Here's how the part is built. I have some questions about the finished solid (model axes, mm). Face numbers are marked on the shaded views. A direction names the side the tool comes from. Coordinates: 2 decimals unless noted, no trailing zeros. Write each loop counter-clockwise with the first axis right and the second up, starting at its lowest first coordinate (ties: lowest second). Pieces come first, ordered by that corner, then holes. Notation, with made-up numbers: (2.5, 58.5) -> (47.5, 58.5) arc R34 cw to (47.5, 90.5) -> close; hole circle Ø8 at (-3, -27.5). An arc over 180 degrees is marked (long way). Put each result on its own line as item: value. Start each with the question number.
Item 1: If we mould it in two halves opening along Y, with no side actions, what happens to the marked faces 6, 7, 8 and 9? For each: released by +Y, released by -Y, zero draft, split by the parting line, or undercut.
Item 2: I need wall thicknesses on line 1 (Y direction, x = -12.75, z = -3.5); line 2 (Y direction, x = -15.75, z = -1.5); line 3 (Z direction, x = -14, y = 3.75). Which ranges of each line are inside material? Lowest first, please. Write a range as [from, to].
Item 3: On a 3-axis mill with a long thin cutter (end or side, diameter ignored), from which of +Z, -Z, +X, -X, +Y, -Y can I reach the whole of each face in a straight line? I mean the marked faces 1, 2, 3, 4 and 5. Say none if no direction works.
Item 4: I want a section at C-C, the plane y = -5.75. List the corners of the cut face in (x, z) for me, then the cut area to 3 significant figures.
Item 5: I want a section at D-D, the plane x = -10.5. List the corners of the cut face in (y, z) for me (3 decimals).
Item 6: I want a section at A-A, the plane x = -15. List the corners of the cut face in (y, z) for me (3 decimals).
Item 7: For pin 1 (0.7 mm diameter, centred on y = -8.5, z = -2.5, fed in from -X); pin 2 (0.5 mm diameter, centred on y = -4.5, z = 3.5, fed in from -X); pin 3 (2 mm diameter, centred on y = 4.5, z = 1, fed in from -X), each with a flat end and sliding along its axis, tell me the tip position at first contact or that it passes through.
Item 8: I want a section at B-B, the plane z = -2.25. List the corners of the cut face in (x, y) for me, then the cut area to 3 significant figures.
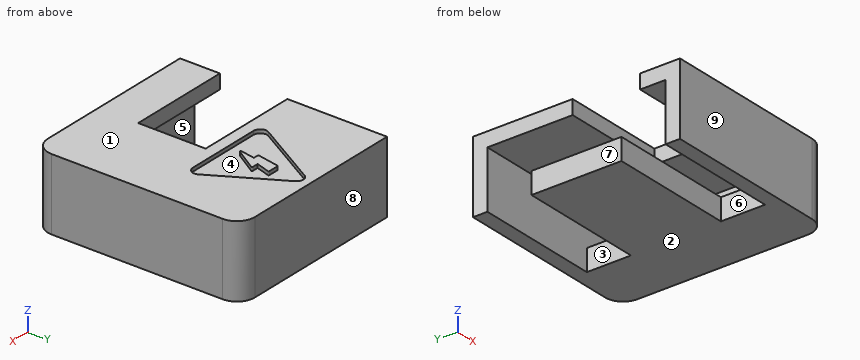
from build123d import *

# Parameters (mm, degrees)
ESQUISSE1_W             = 8
ESQUISSE1_H             = 23
BOSS_EXTRU_1_DEPTH      = 1.6
ESQUISSE2_W             = 2.4
ESQUISSE2_H             = 10
BOSS_EXTRU_2_DEPTH      = 19
ESQUISSE3_W             = 2.4
ESQUISSE3_H             = 19.8
BOSS_EXTRU_3_DEPTH      = 5
ENL_V_MAT_EXTRU_1_REACH = 25.606
ESQUISSE4_W             = 11.5
ESQUISSE4_H             = 7.5
ENL_V_START             = -0.4
ENL_V_MAT_EXTRU_2_DEPTH = 0.4
CONG_1_R                = 2


# Read off the part's stored shape, not the designer's step: Enlèv. mat.-Extru.2
with BuildPart() as part:
    # Esquisse1 → Boss.-Extru.1 (new body)
    with BuildSketch(Plane(origin=(0, 0, 0), x_dir=(0, 0, -1), z_dir=(1, 0, 0))):
        Rectangle(ESQUISSE1_W, ESQUISSE1_H)
    extrude(amount=BOSS_EXTRU_1_DEPTH)

    # Esquisse2 → Boss.-Extru.2 (add)
    with BuildSketch(Plane.ZY):
        Polygon((-4, 11.5), (4, 11.5), (4, -11.5), (-4, -11.5), (-4, -9.9), (2.4, -9.9), (2.4, 9.9), (-4, 9.9), align=None)
        with Locations((-2.8, 0)):
            Rectangle(ESQUISSE2_W, ESQUISSE2_H)
    extrude(amount=BOSS_EXTRU_2_DEPTH)

    # Esquisse3 → Boss.-Extru.3 (add)
    with BuildSketch(Plane.ZY):
        with Locations((-2.8, 0)):
            Rectangle(ESQUISSE3_W, ESQUISSE3_H)
    extrude(amount=BOSS_EXTRU_3_DEPTH)

    # Esquisse4 → Enlèv. mat.-Extru.1 (cut, up to next)
    with BuildSketch(Plane.XY.offset(4), mode=Mode.PRIVATE) as enl_v_mat_extru_1_sk1:
        with Locations((-13.25, -3.325)):
            Rectangle(ESQUISSE4_W, ESQUISSE4_H)
    enl_v_mat_extru_1_tool1 = extrude(enl_v_mat_extru_1_sk1.sketch, amount=-ENL_V_MAT_EXTRU_1_REACH, mode=Mode.PRIVATE) & part.part
    add(enl_v_mat_extru_1_tool1.solids().sort_by_distance((-13.25, -3.325, 4))[0], mode=Mode.SUBTRACT)

    # Enlèv. mat.-Extru.2 outline → Enlèv. mat.-Extru.2 (cut)
    with BuildSketch(Plane.XY.offset(4).offset(ENL_V_START)):
        with BuildLine():
            Line((-12.608271193, 1.69730271), (-4.088687559, 1.69730271))
            add(Edge.make_bspline(
                [(-4.088687559, 1.69730271), (-3.506604225, 1.697303518), (-3.136187559, 2.332303518), (-3.432521215, 2.840303033)],
                knots=[5, 5, 5, 5, 6, 6, 6, 6], degree=3))
            Line((-3.432521215, 2.840303033), (-7.687021295, 10.227470021))
            add(Edge.make_bspline(
                [(-7.687021295, 10.227470021), (-7.983354547, 10.735470041), (-8.713604709, 10.735470041), (-9.009937961, 10.227470021)],
                knots=[1, 1, 1, 1, 2, 2, 2, 2], degree=3))
            Line((-9.009937961, 10.227470021), (-13.275021213, 2.840303033))
            add(Edge.make_bspline(
                [(-13.275021213, 2.840303033), (-13.571354541, 2.33230271), (-13.200937899, 1.69730271), (-12.608271193, 1.69730271)],
                knots=[3, 3, 3, 3, 4, 4, 4, 4], degree=3))
        make_face()
        with BuildLine():
            add(Edge.make_bspline(
                [(-7.380104467, 5.570803355), (-7.337771376, 5.623720022), (-7.380104467, 5.708386608), (-7.454188284, 5.708387012)],
                knots=[11, 11, 11, 11, 12, 12, 12, 12], degree=3))
            Line((-7.380104467, 5.570803355), (-8.9146878, 3.115470345))
            add(Edge.make_bspline(
                [(-9.0734378, 3.178970184), (-9.094604547, 3.083720023), (-8.967604466, 3.030803356), (-8.9146878, 3.115470345)],
                knots=[1, 1, 1, 1, 2, 2, 2, 2], degree=3))
            Line((-9.0734378, 3.178970184), (-8.787687719, 4.766470184))
            Line((-8.787687719, 4.766470184), (-9.306271214, 4.766470184))
            add(Edge.make_bspline(
                [(-9.390937799, 4.872303517), (-9.401521375, 4.81938685), (-9.35918788, 4.766470184), (-9.306271214, 4.766470184)],
                knots=[4, 4, 4, 4, 5, 5, 5, 5], degree=3))
            Line((-9.390937799, 4.872303517), (-8.957021294, 7.253553516))
            add(Edge.make_bspline(
                [(-8.872354708, 7.32763693), (-8.9146878, 7.32763693), (-8.946438123, 7.295887011), (-8.957021294, 7.253553516)],
                knots=[6, 6, 6, 6, 7, 7, 7, 7], degree=3))
            Line((-8.872354708, 7.32763693), (-7.739937961, 7.32763693))
            add(Edge.make_bspline(
                [(-7.655271375, 7.211220425), (-7.634104628, 7.274720264), (-7.676438123, 7.32763693), (-7.739937961, 7.32763693)],
                knots=[8, 8, 8, 8, 9, 9, 9, 9], degree=3))
            Line((-7.655271375, 7.211220425), (-8.120938204, 5.708387012))
            Line((-8.120938204, 5.708387012), (-7.454188284, 5.708387012))
        make_face(mode=Mode.SUBTRACT)
    extrude(amount=ENL_V_MAT_EXTRU_2_DEPTH, mode=Mode.SUBTRACT)

    # Congé1
    cong_1_edges = [part.edges().sort_by_distance(p)[0] for p in [
        (1.6, -11.5, 0),
        (1.6, 11.5, 0),
    ]]
    fillet(cong_1_edges, radius=CONG_1_R)


solid = part.part
Calculated:
1. face 6: undercut
1. face 7: zero draft
1. face 8: released by +Y
1. face 9: released by -Y
2. line 1: y = [-11.5, -9.9], [-5, 5], [9.9, 11.5]
2. line 2: y = [-11.5, -9.9], [9.9, 11.5]
2. line 3: z = [-4, -1.6], [2.4, 4]
3. face 1: +Z, +X, -X, +Y, -Y
3. face 2: -Z, +X, -X, +Y, -Y
3. face 3: -Z, -X
3. face 4: +Z
3. face 5: -X
4. outline: (-7.5, 2.4) -> (0, 2.4) -> (0, -1.6) -> (-5, -1.6) -> (-5, -4) -> (1.6, -4) -> (1.6, 4) -> (-7.5, 4) -> close
4. area: 36.8 mm2
5. outline: (-11.5, -4) -> (-9.9, -4) -> (-9.9, 2.4) -> (-7.075, 2.4) -> (-7.075, 4) -> (-11.5, 4) -> close; (-5, -4) -> (5, -4) -> (5, -1.6) -> (-5, -1.6) -> close; (0.425, 2.4) -> (9.9, 2.4) -> (9.9, -4) -> (11.5, -4) -> (11.5, 4) -> (7.647, 4) -> (7.647, 3.6) -> (1.697, 3.6) -> (1.697, 4) -> (0.425, 4) -> close
6. outline: (-11.5, -4) -> (-9.9, -4) -> (-9.9, 2.4) -> (-7.075, 2.4) -> (-7.075, 4) -> (-11.5, 4) -> close; (-5, -4) -> (5, -4) -> (5, -1.6) -> (-5, -1.6) -> close; (0.425, 2.4) -> (9.9, 2.4) -> (9.9, -4) -> (11.5, -4) -> (11.5, 4) -> (0.425, 4) -> close
7. pin 1: stops at x = -5
7. pin 2: stops at x = -7.5
7. pin 3: stops at x = 0
8. outline: (-19, -11.5) -> (-0.4, -11.5) arc R2 ccw to (1.6, -9.5) -> (1.6, 9.5) arc R2 ccw to (-0.4, 11.5) -> (-19, 11.5) -> (-19, 9.9) -> (-5, 9.9) -> (-5, 5) -> (-19, 5) -> (-19, -5) -> (-5, -5) -> (-5, -9.9) -> (-19, -9.9) -> close
8. area: 335 mm2
